Part model, mm, in its own coordinate system. Face numbers are marked on the shaded views. A direction names the side the tool comes from. Give positions to 0.01 mm unless a question says otherwise; leave off trailing zeros. Loops run counter-clockwise (first coordinate to the right, second up) from the corner with the lowest first, then second, coordinate; pieces in that order, holes last. Notation, with made-up numbers: (-9, -39.75) -> (30, -39.75) arc R25 cw to (30, -2.75) -> close; hole circle Ø6 at (-5.75, -30.5). An arc over 180 degrees is marked (long way). One line per question, with ' | ' between items.
```python
from build123d import *

# Parameters (mm, degrees)
SKETCH3_W           = 52
SKETCH3_H           = 25
BOSS_EXTRUDE3_DEPTH = 2
SKETCH4_W           = 25
SKETCH4_H           = 14.5
BOSS_EXTRUDE4_DEPTH = 2
BOSS_EXTRUDE5_DEPTH = 2
SKETCH6_R           = 1.65
CUT_EXTRUDE1_DEPTH  = 2
SKETCH7_R           = 3.75
SKETCH7_R_2         = 1.65
CUT_EXTRUDE2_DEPTH  = 2
FILLET1_R           = 1


with BuildPart() as part:
    # Sketch3 → Boss-Extrude3 (new body)
    with BuildSketch(Plane(origin=(0, 0, 0), x_dir=(1, 0, 0), z_dir=(0, 1, 0))):
        with Locations((26, 12.5)):
            Rectangle(SKETCH3_W, SKETCH3_H)
    extrude(amount=BOSS_EXTRUDE3_DEPTH)

    # Sketch4 → Boss-Extrude4 (add)
    with BuildSketch(Plane(origin=(0, 0, 0), x_dir=(0, 0, -1), z_dir=(1, 0, 0))):
        with Locations((12.5, 7.25)):
            Rectangle(SKETCH4_W, SKETCH4_H)
    extrude(amount=BOSS_EXTRUDE4_DEPTH)

    # Sketch5 → Boss-Extrude5 (add)
    with BuildSketch(Plane.ZY):
        with BuildLine():
            Line((-25, 0), (0, 0))
            Line((0, 0), (0, 14.5))
            ThreePointArc((0, 14.5), (-12.5, 27), (-25, 14.5))
            Line((-25, 14.5), (-25, 0))
        make_face()
    extrude(amount=-BOSS_EXTRUDE5_DEPTH)

    # Sketch6 → Cut-Extrude1 (cut)
    with BuildSketch(Plane(origin=(0, 2, 0), x_dir=(1, 0, 0), z_dir=(0, 1, 0))):
        with Locations(Location((12, 12.5, 0), (0, 0, 270))):
            Circle(SKETCH6_R)
        with Locations(Location((22, 12.5, 0), (0, 0, 270))):
            Circle(SKETCH6_R)
        with Locations(Location((32, 12.5, 0), (0, 0, 270))):
            Circle(SKETCH6_R)
        with Locations(Location((42, 12.5, 0), (0, 0, 270))):
            Circle(SKETCH6_R)
    extrude(amount=-CUT_EXTRUDE1_DEPTH, mode=Mode.SUBTRACT)

    # Sketch7 → Cut-Extrude2 (cut)
    with BuildSketch(Plane.ZY):
        with Locations((-12.5, 14.5)):
            Circle(SKETCH7_R)
        with Locations((-21, 14.5)):
            Circle(SKETCH7_R_2)
        with Locations((-4, 14.5)):
            Circle(SKETCH7_R_2)
        with Locations((-12.5, 6)):
            Circle(SKETCH7_R_2)
        with Locations((-12.5, 23)):
            Circle(SKETCH7_R_2)
    extrude(amount=-CUT_EXTRUDE2_DEPTH, mode=Mode.SUBTRACT)

    # Fillet1
    fillet1_edges = [part.edges().sort_by_distance(p)[0] for p in [
        (2, 2, -12.5),
        (0, 0, -12.5),
        (52, 1, -25),
        (52, 1, 0),
    ]]
    fillet(fillet1_edges, radius=FILLET1_R)


solid = part.part
```
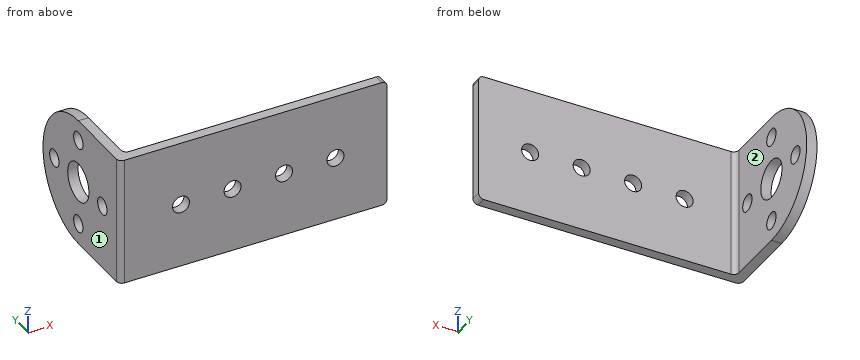
1) Saw through at A-A (x = 12). Give the cut face in (y, z), and give its area (3 significant figures).
Found:
outline: (0, -25) -> (2, -25) -> (2, -14.15) -> (0, -14.15) -> close; (0, -10.85) -> (2, -10.85) -> (2, 0) -> (0, 0) -> close | area: 43.4 mm2
2) Drill centre lines: line 1 (X direction, y = 0.7, z = -12.5); line 2 (Y direction, x = 6.5, z = -17.25). Where is each one in solid material? Low to high.
Found:
line 1: 0.05 to 10.35, 13.65 to 20.35, 23.65 to 30.35, 33.65 to 40.35, 43.65 to 52 | line 2: 0 to 2
3) Pin check, flat tips, straight feed: P1, Ø12, axis at y = 18, z = -7.5, coming from the +X side; P2, Ø4, axis at x = 42, z = -12.5, coming from the +Y side. Stop position of each tip, or through.
Found:
P1: x = 2 | P2: y = 2
4) Saw through at D-D (z = -12.5). State how many separate pieces and enclosed holes the cut face has, and give its area (3 significant figures).
Found:
separate pieces: 8 | enclosed holes: 0 | area: 99.4 mm2
5) Saw through at B-B (z = -22). Give the cut face in (x, y).
Found:
outline: (0, 1) arc R1 ccw to (1, 0) -> (52, 0) -> (52, 2) -> (3, 2) arc R1 cw to (2, 3) -> (2, 13.19) -> (0, 13.19) -> close; (0, 15.81) -> (2, 15.81) -> (2, 22.62) -> (0, 22.62) -> close
6) Tool access for the marked faces 1 and 2: list every direction of +Z, -Z, +X, -X, +Y, -Y with a clear straight run to the whole face (end or side of a thin tool).
Found:
face 1: +Z, -Z, -X, +Y, -Y | face 2: +Z, -Z, +X, +Y
7) Saw through at C-C (y = 12). Give the cut face in (x, z).
Found:
outline: (0, -25) -> (2, -25) -> (2, -15.3) -> (0, -15.3) -> close; (0, -9.7) -> (2, -9.7) -> (2, 0) -> (0, 0) -> close
